Check sheet for the modelled part. Datum: model origin and axes. Units: mm. A direction names the side the tool comes from. Give positions to 0.01 mm unless a question says otherwise; leave off trailing zeros. Write each loop counter-clockwise with the first axis right and the second up, starting at its lowest first coordinate (ties: lowest second). Pieces come first, ordered by that corner, then holes. Notation, with made-up numbers: M -37.5,17.5 L -6.5,17.5 A11 cw -6.5,38.5 Z; hole C 61.5,23.5 d2. An arc over 180 degrees is marked long. Write item = value, one per line. Start each with the question number.
1) Go/stop test with flat-tipped pins: pin 1 (1.1 mm diameter, centred on y = -12.5, z = -2, fed in from -X); pin 2 (5 mm diameter, centred on x = 162.5, y = 12, fed in from -Z); pin 3 (1.1 mm diameter, centred on x = 177.5, z = -2, fed in from +Y); pin 4 (1.8 mm diameter, centred on x = -9.5, z = -2, fed in from -Y). Record where each tip stops, or that it passes through.
2) Cross-section at D-D, the plane x = 48. Record the cut outline in (y, z).
3) Access from +Z, -Z, +X, -X, +Y, -Y to the whole of each face (thin tool, end or side, straight path). Record for faces 1 (the flat face through (188, 40, -2)), 2 (the flat face through (188, 24, -2)), 3 (the flat face through (-18, 40, -2)), 4 (the flat face through (50, -10, -2)), 5 (the flat face through (-18, 14, -2)).
4) Cross-section at B-B, the plane y = 16.5. Record the cut outline in (x, z), plus the area to 3 significant figures.
5) Scan lines: line 1 along Y through (x, z) = (128.2, -2.85); line 2 along X through (y, z) = (21, -1.3); line 3 along Y through (x, z) = (7.5, -2.7). Record each from-to range of solid material in increasing order. Write a range as [from, to].
6) Cross-section at C-C, the plane z = -1.55. Give the number of separate pieces and of enclosed holes in the cut face, plus the area to 3 significant figures.
7) Mould release check, pull along X, two halves, no side actions. Record for faces 6 (the flat face through (166, -12, -2)), 7 (the flat face through (142, 50, -2)), 8 (the flat face through (176, 48, -2)): released by +X, released by -X, zero draft, split by the parting line, or undercut.
8) Cross-section at A-A, the plane x = 137. Record the cut outline in (y, z).
```python
from build123d import *

# Parameters (mm, degrees)
SKETCH_1_W             = 170
SKETCH_1_H             = 48
SKETCH_1_R             = 2
SKETCH_1_R_2           = 6.5
SKETCH_1_R_3           = 1.6
SM_BASE_FLANGE_1_DEPTH = 3.6
SKETCH_7_W             = 16
SKETCH_7_H             = 48
EXTRUDE_1_DEPTH        = 3.6
SKETCH_8_W             = 202
SKETCH_8_H             = 10
EXTRUDE_2_DEPTH        = 3.6
SKETCH_9_W             = 3.6
SKETCH_9_H             = 16
SKETCH_9_W_2           = 24
SKETCH_9_H_2           = 3.6
SKETCH_9_W_3           = 26
EXTRUDE_3_DEPTH        = 3.6


# Sheet-metal steps are written as plain solids
with BuildPart() as part:
    # Sketch 1 → Базовая кромка1 (new body)
    with BuildSketch(Plane.XY):
        with Locations((85, 24)):
            Rectangle(SKETCH_1_W, SKETCH_1_H)
        with Locations((137, 12)):
            Circle(SKETCH_1_R, mode=Mode.SUBTRACT)
        with Locations((33, 12)):
            Circle(SKETCH_1_R, mode=Mode.SUBTRACT)
        with Locations((148.55, 12)):
            Circle(SKETCH_1_R_2, mode=Mode.SUBTRACT)
        with Locations((21.45, 12)):
            Circle(SKETCH_1_R_2, mode=Mode.SUBTRACT)
        with Locations((128.2, 20.65)):
            Circle(SKETCH_1_R_3, mode=Mode.SUBTRACT)
        with Locations((128.2, 3.35)):
            Circle(SKETCH_1_R_3, mode=Mode.SUBTRACT)
        with Locations((41.8, 20.65)):
            Circle(SKETCH_1_R_3, mode=Mode.SUBTRACT)
        with Locations((41.8, 3.35)):
            Circle(SKETCH_1_R_3, mode=Mode.SUBTRACT)
        with Locations((162.5, 12)):
            Circle(SKETCH_1_R_3, mode=Mode.SUBTRACT)
        with Locations((7.5, 12)):
            Circle(SKETCH_1_R_3, mode=Mode.SUBTRACT)
    extrude(amount=-SM_BASE_FLANGE_1_DEPTH)

    # Эскиз7 → Бобышка-Вытянуть1 (add)
    with BuildSketch(Plane(origin=(0, 0, -3.6), x_dir=(-1, 0, 0), z_dir=(0, 0, -1))):
        with Locations((-178, 24)):
            Rectangle(SKETCH_7_W, SKETCH_7_H)
        with Locations((8, 24)):
            Rectangle(SKETCH_7_W, SKETCH_7_H)
    extrude(amount=-EXTRUDE_1_DEPTH)

    # Эскиз8 → Бобышка-Вытянуть2 (add)
    with BuildSketch(Plane(origin=(0, 0, -3.6), x_dir=(-1, 0, 0), z_dir=(0, 0, -1))):
        with Locations((-85, -5)):
            Rectangle(SKETCH_8_W, SKETCH_8_H)
    extrude(amount=-EXTRUDE_2_DEPTH)

    # Эскиз9 → Бобышка-Вытянуть3 (add)
    with BuildSketch(Plane(origin=(0, 0, -3.6), x_dir=(-1, 0, 0), z_dir=(0, 0, -1))):
        with Locations((-187.8, 32)):
            Rectangle(SKETCH_9_W, SKETCH_9_H)
        with Locations((-187.8, 6)):
            Rectangle(SKETCH_9_W, SKETCH_9_H)
        with Locations((-154, 49.8)):
            Rectangle(SKETCH_9_W_2, SKETCH_9_H_2)
        with Locations((-85, 49.8)):
            Rectangle(SKETCH_9_W_3, SKETCH_9_H_2)
        with Locations((-16, 49.8)):
            Rectangle(SKETCH_9_W_2, SKETCH_9_H_2)
        with Locations((17.8, 32)):
            Rectangle(SKETCH_9_W, SKETCH_9_H)
        with Locations((17.8, 6)):
            Rectangle(SKETCH_9_W, SKETCH_9_H)
        with Locations((-16, -11.8)):
            Rectangle(SKETCH_9_W_2, SKETCH_9_H_2)
        with Locations((-85, -11.8)):
            Rectangle(SKETCH_9_W_3, SKETCH_9_H_2)
        with Locations((-154, -11.8)):
            Rectangle(SKETCH_9_W_2, SKETCH_9_H_2)
    extrude(amount=-EXTRUDE_3_DEPTH)


solid = part.part
```
Reply:
q1.pin_1 = 4
q1.pin_2 = -3.6
q1.pin_3 = 48
q1.pin_4 = -10
q2.outline = M -10,-3.6 L 48,-3.6 L 48,0 L -10,0 Z
q3.face_1 = +Z, -Z, +X, +Y
q3.face_2 = +Z, -Z, +X
q3.face_3 = +Z, -Z, -X, +Y
q3.face_4 = +Z, -Z, -Y
q3.face_5 = +Z, -Z, -X
q4.outline = M -16,-3.6 L 16.76,-3.6 L 16.76,0 L -16,0 Z; M 26.14,-3.6 L 143.86,-3.6 L 143.86,0 L 26.14,0 Z; M 153.24,-3.6 L 186,-3.6 L 186,0 L 153.24,0 Z
q4.area = 660 mm2
q5.line_1 = [-10, 1.75], [4.95, 19.05], [22.25, 48]
q5.line_2 = [-16, 40.24], [43.36, 126.64], [129.76, 186]
q5.line_3 = [-13.6, 10.4], [13.6, 51.6]
q6.separate_pieces = 1
q6.enclosed_holes = 10
q6.area = 12,100 mm2
q7.face_6 = released by +X
q7.face_7 = undercut
q7.face_8 = zero draft
q8.outline = M -10,-3.6 L 10,-3.6 L 10,0 L -10,0 Z; M 14,-3.6 L 48,-3.6 L 48,0 L 14,0 Z
